Input: part model. Units: mm. Frame: model coordinates. A direction names the side the tool comes from. Round coordinates to 2 decimals unless told otherwise and drop trailing zeros. Loops run counter-clockwise (first coordinate to the right, second up) from the corner with the lowest first, then second, coordinate; pieces in that order, holes last. Notation, with made-up numbers: (32, -25.75) - (62, -25.75) arc R37 ccw to (62, 11.25) - close; hole circle Ø1 at (44, 73.5). An arc over 180 degrees is marked (long way). Write each question's results on one line, items separated by ' | '.
from build123d import *

# Parameters (mm, degrees)
BOSS_EXTRU_1_DEPTH      = 20
ESQUISSE2_R             = 1.5
ENL_V_MAT_EXTRU_1_DEPTH = 20
ESQUISSE3_R             = 1.5
ENL_V_MAT_EXTRU_2_DEPTH = 20
CHANFREIN1_SIZE         = 2.5
CONG_2_R                = 1


with BuildPart() as part:
    # Esquisse1 → Boss.-Extru.1 (new body)
    with BuildSketch(Plane.XY):
        Polygon((23, 0), (0, 0), (0, 23), (3, 23), (3, 3), (23, 3), align=None)
    extrude(amount=BOSS_EXTRU_1_DEPTH)

    # Esquisse2 → Enlèv. mat.-Extru.1 (cut)
    with BuildSketch(Plane(origin=(0, 3, 0), x_dir=(1, 0, 0), z_dir=(0, 1, 0))):
        with Locations((8, -15)):
            Circle(ESQUISSE2_R)
        with Locations((18, -15)):
            Circle(ESQUISSE2_R)
        with Locations((18, -5)):
            Circle(ESQUISSE2_R)
        with Locations((8, -5)):
            Circle(ESQUISSE2_R)
    extrude(amount=-ENL_V_MAT_EXTRU_1_DEPTH, mode=Mode.SUBTRACT)

    # Esquisse3 → Enlèv. mat.-Extru.2 (cut)
    with BuildSketch(Plane(origin=(3, 0, 0), x_dir=(0, 0, -1), z_dir=(1, 0, 0))):
        with Locations((-15, 18)):
            Circle(ESQUISSE3_R)
        with Locations((-5, 18)):
            Circle(ESQUISSE3_R)
        with Locations((-5, 8)):
            Circle(ESQUISSE3_R)
        with Locations((-15, 8)):
            Circle(ESQUISSE3_R)
    extrude(amount=-ENL_V_MAT_EXTRU_2_DEPTH, mode=Mode.SUBTRACT)

    # Chanfrein1
    chanfrein1_edges = [part.edges().sort_by_distance(p)[0] for p in [
        (3, 3, 10),
    ]]
    chamfer(chanfrein1_edges, length=CHANFREIN1_SIZE)

    # Congé2
    cong_2_edges = [part.edges().sort_by_distance(p)[0] for p in [
        (23, 0, 10),
        (0, 0, 10),
        (0, 23, 10),
        (3, 23, 10),
        (23, 3, 10),
        (3, 5.5, 10),
        (5.5, 3, 10),
    ]]
    fillet(cong_2_edges, radius=CONG_2_R)


solid = part.part
1. Mould query, pull axis X, two halves, no side actions, for faces 3 (the cylindrical face through (6.89, 1.52, 3.99)), 4 (the cylindrical face through (1.52, 8.07, 16.5)), 5 (the flat face through (0, 11, 10)). Classes: pulls with the +X half, pulls with the -X half, needs draft (parallel to the pull), parting line crosses it, or undercut.
Answer:
face 3: undercut | face 4: needs draft | face 5: pulls with the -X half
2. Section query A-A, the plane x = 18. Output: boundary loops of the cut face in (y, z).
Answer:
outline: (0, 0) - (3, 0) - (3, 3.5) - (0, 3.5) - close; (0, 6.5) - (3, 6.5) - (3, 13.5) - (0, 13.5) - close; (0, 16.5) - (3, 16.5) - (3, 20) - (0, 20) - close
3. Line query: line 1 (Y direction, x = 1.35, z = 15); line 2 (Z direction, x = 18, y = 2.15). Output: solid intervals per line, ascending. Write a range as [from, to].
Answer:
line 1: [0, 6.5], [9.5, 16.5], [19.5, 23] | line 2: [0, 3.5], [6.5, 13.5], [16.5, 20]
4. Section query B-B, the plane z = 5. Count the separate pieces of the cut face and the enclosed holes in it, plus the area to 3 significant figures.
Answer:
separate pieces: 5 | enclosed holes: 0 | area: 95.1 mm^2
5. Set-up query: faces 1 (the flat face through (14, 3, 10)), 2 (the cylindrical face through (16.5, 1.52, 14.93)). Return all of +Z, -Z, +X, -X, +Y, -Y with unobstructed straight access to the full face (end or side cutting, diameter ignored); none if empty.
Answer:
face 1: +Z, -Z, +X, +Y | face 2: +Y, -Y
6. Contact query for flat-ended pins moving along their axis: pin 1 (2.5 mm diameter, centred on x = 8, z = 5, fed in from -Y); pin 2 (5 mm diameter, centred on y = 15.5, z = 5, fed in from +X); pin 3 (3.5 mm diameter, centred on x = 18, z = 5, fed in from +Y); pin 4 (10 mm diameter, centred on y = 8.5, z = 16, fed in from +X). Output: stop coordinate, or through.
Answer:
pin 1: through | pin 2: x = 3 | pin 3: y = 3 | pin 4: x = 5
7. Section query D-D, the plane z = 9. Output: boundary loops of the cut face in (x, y), plus the area to 3 significant figures.
Answer:
outline: (0, 1) arc R1 ccw to (1, 0) - (22, 0) arc R1 ccw to (23, 1) - (23, 2) arc R1 ccw to (22, 3) - (5.91, 3) arc R1 cw to (5.21, 3.29) - (3.29, 5.21) arc R1 cw to (3, 5.91) - (3, 22) arc R1 ccw to (2, 23) - (1, 23) arc R1 ccw to (0, 22) - close | area: 131 mm^2
